from build123d import *

# Parameters (mm, degrees)
SKETCH001_W                      = 6.7
SKETCH001_H                      = 125
PAD004_DEPTH                     = 70
SKETCH001002002010004010_R       = 12
SKETCH001002002010004010_R_2     = 11
SKETCH001002002010004010_R_3     = 3.264
SKETCH001002002010004010_R_4     = 1.5875
POCKET008_DEPTH                  = 293.545139
POCKET009_DEPTH                  = 293.545139
SKETCH001002002010004011001005_W = 6.7
SKETCH001002002010004011001005_H = 6.7818
PAD005_DEPTH                     = 6.7


with BuildPart() as part:
    # Sketch001 → Pad004 (new body)
    with BuildSketch(Plane.XY.offset(3.35)):
        with Locations((4.7, 0)):
            Rectangle(SKETCH001_W, SKETCH001_H)
    extrude(amount=PAD004_DEPTH)

    # Sketch001002002010004010 → Pocket008 (cut, through all)
    with BuildSketch(Plane(origin=(1.35, 0, 3.35), x_dir=(0, -1, 0), z_dir=(-1, 0, 0))):
        with Locations((-44, 35)):
            Circle(SKETCH001002002010004010_R)
        with Locations((0, 47.514)):
            Circle(SKETCH001002002010004010_R_2)
        with Locations((-37.788344, 58.18222)):
            Circle(SKETCH001002002010004010_R_3)
        with Locations((-50.211656, 11.81778)):
            Circle(SKETCH001002002010004010_R_3)
        with Locations((-15.494, 63.008)):
            Circle(SKETCH001002002010004010_R_4)
        with Locations((-15.494, 32.02)):
            Circle(SKETCH001002002010004010_R_4)
    pocket008 = extrude(amount=-POCKET008_DEPTH, mode=Mode.SUBTRACT)

    # Mirrored: Pocket008 across Sketch001002002010004010 V_Axis
    add(pocket008.mirror(Plane(origin=(1.35, 0, 3.35), x_dir=(-1, 0, 0), z_dir=(0, -1, 0))), mode=Mode.SUBTRACT)

    # Sketch001002002010004011001004 → Pocket009 (cut, through all)
    with BuildSketch(Plane(origin=(1.35, 0, 3.35), x_dir=(0, -1, 0), z_dir=(-1, 0, 0))):
        Polygon((-37.77, -1e-06), (-37.770004, 12.079999), (-39.925004, 12.079998), (-39.925006, 18.579998), (-37.770006, 18.579999), (-37.770007, 22.279999), (-33.350007, 22.28), (-33.350006, 18.58), (-31.195006, 18.580001), (-31.195004, 12.080001), (-33.350004, 12.08), (-33.35, 0), (-35.56, -1e-06), align=None)
    pocket009 = extrude(amount=-POCKET009_DEPTH, mode=Mode.SUBTRACT)

    # Mirrored001: Pocket009 across Sketch001002002010004011001004 V_Axis
    add(pocket009.mirror(Plane(origin=(1.35, 0, 3.35), x_dir=(-1, 0, 0), z_dir=(0, -1, 0))), mode=Mode.SUBTRACT)

    # Sketch001002002010004011001005 → Pad005 (new body)
    with BuildSketch(Plane(origin=(0, 0, 3.35), x_dir=(1, 0, 0), z_dir=(0, 0, -1))):
        with Locations((4.7, 21.1709)):
            Rectangle(SKETCH001002002010004011001005_W, SKETCH001002002010004011001005_H)
    pad005 = extrude(amount=PAD005_DEPTH)

    # Mirrored002: Pad005 across Sketch001002002010004011001005 H_Axis
    add(pad005.mirror(Plane(origin=(0, 0, 3.35), x_dir=(0, 0, -1), z_dir=(0, -1, 0))))


solid = part.part
For this review, take the finished solid that the model builds, in its own axes (mm). A direction names the side the tool comes from. Coordinates: 2 decimals unless noted, no trailing zeros. Loops run counter-clockwise (first coordinate to the right, second up) from the corner with the lowest first, then second, coordinate; pieces in that order, holes last. Notation, with made-up numbers: (-2.75, -14.5) - (11.25, -14.5) arc R26 cw to (11.25, 15.5) - close; hole circle Ø1 at (35, 52). An arc over 180 degrees is marked (long way). Use a Markdown table: item, result. Add a question column.
Item 1: We need section B-B (z = 38.35). Give the boundary of the cut face in (x, y).
Item 2: We need section D-D (y = 0). Give the boundary of the cut face in (x, z).
Item 3: We need section C-C (z = 13.5). Give the boundary of the cut face in (x, y).
Item 4: Tool access review of faces 5 (the face through (5, 39.925, 19)), 6 (the face through (5, 29, 3.35)), 7 (the face through (5, -50, 3.35)), 8 (the face through (5, 37.77, 24)): name each direction out of +Z, -Z, +X, -X, +Y, -Y from which nothing blocks a thin tool from reaching the whole face with its end or side.
Item 5: Mouldability with a two-part tool opening along Y and no side actions: class faces 1 (the face through (5, -37.77, 24)), 2 (the face through (5, 62.5, 38)), 3 (the face through (5, -24.562, 0)), 4 (the face through (5, 1, 73.35)) as pulls with the +Y half, pulls with the -Y half, needs draft (parallel to the pull), parting line crosses it, or undercut.
Item 6: Insertion check: pin 1 Ø2 at (x, y) = (6.5, -29) entering from -Z; pin 2 Ø2 at (x, z) = (3.5, 0) entering from +Y; pin 3 Ø3 at (y, z) = (15.494, 66.358) entering from +X. Each pin has a flat end and moves straight along its axis. Give the tip position at first contact, or say it passes through.
Item 7: For line 1 (Y direction, x = 7.25, z = 20.5) (3 decimals); line 2 (Y direction, x = 5.5, z = 22.5); line 3 (Y direction, x = 6.25, z = 15), list the stretches that pass through material, from the lowest coordinate up.
Item 8: We need section A-A (y = 44). Give the boundary of the cut face in (x, z).
Results list:
| question | item | result |
|---|---|---|
| 1 | outline | (1.35, -62.5) - (8.05, -62.5) - (8.05, -56) - (1.35, -56) - close; (1.35, -32) - (8.05, -32) - (8.05, 32) - (1.35, 32) - close; (1.35, 56) - (8.05, 56) - (8.05, 62.5) - (1.35, 62.5) - close |
| 2 | outline | (1.35, 3.35) - (8.05, 3.35) - (8.05, 39.86) - (1.35, 39.86) - close; (1.35, 61.86) - (8.05, 61.86) - (8.05, 73.35) - (1.35, 73.35) - close |
| 3 | outline | (1.35, -62.5) - (8.05, -62.5) - (8.05, -53.02) - (1.35, -53.02) - close; (1.35, -47.41) - (8.05, -47.41) - (8.05, -37.77) - (1.35, -37.77) - close; (1.35, -33.35) - (8.05, -33.35) - (8.05, 33.35) - (1.35, 33.35) - close; (1.35, 37.77) - (8.05, 37.77) - (8.05, 47.41) - (1.35, 47.41) - close; (1.35, 53.02) - (8.05, 53.02) - (8.05, 62.5) - (1.35, 62.5) - close |
| 4 | face 5 | +X, -X |
| 4 | face 6 | -Z, +X, -X, +Y |
| 4 | face 7 | -Z, +X, -X, -Y |
| 4 | face 8 | -Z, +X, -X |
| 5 | face 1 | undercut |
| 5 | face 2 | pulls with the +Y half |
| 5 | face 3 | pulls with the -Y half |
| 5 | face 4 | needs draft |
| 6 | pin 1 | stops at z = 3.35 |
| 6 | pin 2 | stops at y = 24.56 |
| 6 | pin 3 | passes through |
| 7 | line 1 | y = -62.5 to -39.925, -31.195 to 31.195, 39.925 to 62.5 |
| 7 | line 2 | y = -62.5 to -37.77, -33.35 to 33.35, 37.77 to 62.5 |
| 7 | line 3 | y = -62.5 to -53.47, -46.95 to -37.77, -33.35 to 33.35, 37.77 to 46.95, 53.47 to 62.5 |
| 8 | outline | (1.35, 3.35) - (8.05, 3.35) - (8.05, 26.35) - (1.35, 26.35) - close; (1.35, 50.35) - (8.05, 50.35) - (8.05, 73.35) - (1.35, 73.35) - close |
